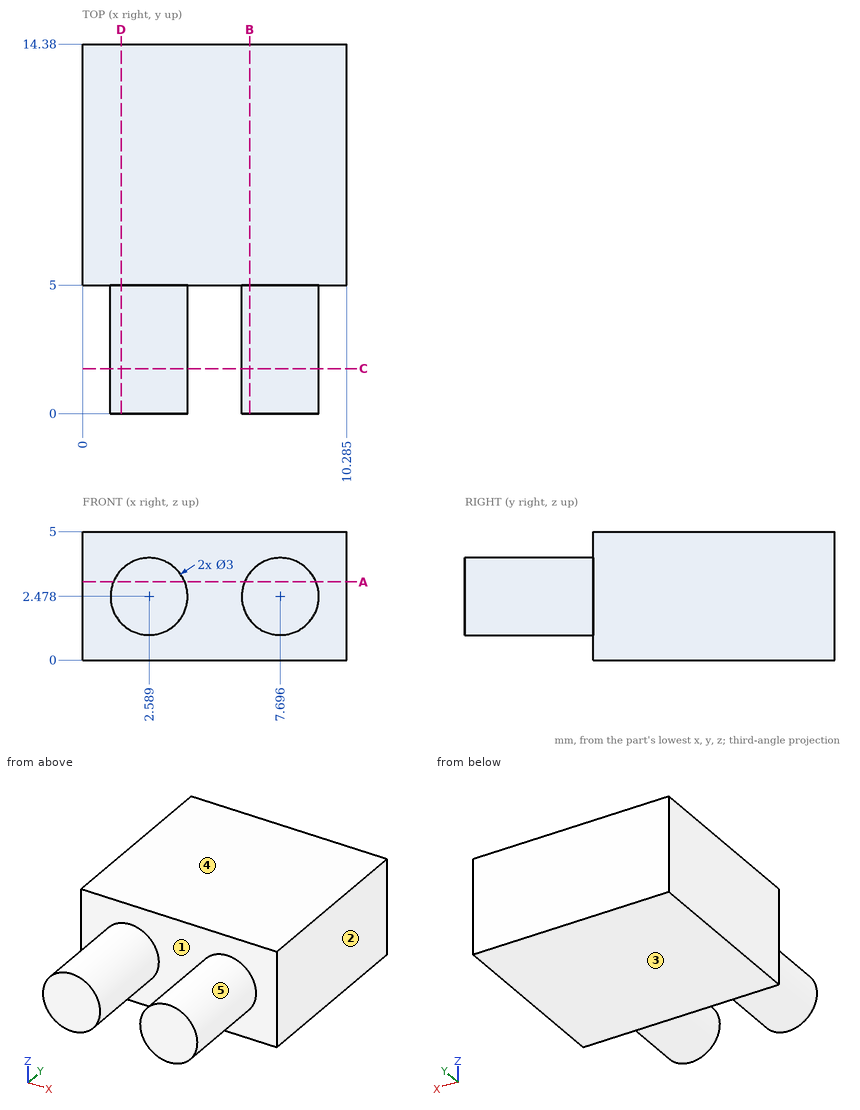
Could you check a few things on this drawing? It's one solid part, dimensions in mm from its lowest x, y, z. A direction names the side the tool comes from. Coordinates: 2 decimals unless noted, no trailing zeros. Loops run counter-clockwise (first coordinate to the right, second up) from the corner with the lowest first, then second, coordinate; pieces in that order, holes last. Notation, with made-up numbers: (16, 35.5) - (57, 35.5) arc R23 ccw to (57, 43.5) - close; hole circle Ø3 at (31, 59.25). An arc over 180 degrees is marked (long way). Return JSON: item names as keys, results as strings. Group by question number.
Item 1: If we section it at D-D on x = 1.5: Write out the boundary of the cut face in (y, z).
Item 2: I need wall thicknesses on line 1 (Y direction, x = 4.75, z = 3); line 2 (X direction, y = 4.25, z = 3.2) (1 decimal); line 3 (Z direction, x = 2, y = 4). Which ranges of each line are inside material? Lowest first, please. Write a range as from..to.
Item 3: If we section it at C-C on y = 1.75: Write out the boundary of the cut face in (x, z) (1 decimal).
Item 4: If we section it at B-B on x = 6.5: Write out the boundary of the cut face in (y, z).
Item 5: If we section it at A-A on z = 3.05: Write out the boundary of the cut face in (x, y) (1 decimal).
Item 6: On a 3-axis mill with a long thin cutter (end or side, diameter ignored), from which of +Z, -Z, +X, -X, +Y, -Y can I reach the whole of each face in a straight line? I mean the marked faces 4 and 5. Say none if no direction works.
Item 7: We'd pull the mould along X, two halves only. Please class the marked faces 1, 2 and 3: +X half, -X half, draft (parallel to the pull), parting line (faces both ways), or undercut.
Calculated:
{
 "1": {"outline": "(0, 1.45) - (5, 1.45) - (5, 0) - (14.38, 0) - (14.38, 5) - (5, 5) - (5, 3.51) - (0, 3.51) - close"},
 "2": {"line 1": "y = 5..14.38", "line 2": "x = 1.3..3.9, 6.4..9", "line 3": "z = 1.1..3.86"},
 "3": {"outline": "circle Ø3 at (2.6, 2.5); circle Ø3 at (7.7, 2.5)"},
 "4": {"outline": "(0, 1.57) - (5, 1.57) - (5, 0) - (14.38, 0) - (14.38, 5) - (5, 5) - (5, 3.38) - (0, 3.38) - close"},
 "5": {"outline": "(0, 5) - (1.2, 5) - (1.2, 0) - (4, 0) - (4, 5) - (6.3, 5) - (6.3, 0) - (9.1, 0) - (9.1, 5) - (10.3, 5) - (10.3, 14.4) - (0, 14.4) - close"},
 "6": {"face 4": "+Z, +X, -X, +Y, -Y", "face 5": "-Y"},
 "7": {"face 1": "undercut", "face 2": "+X half", "face 3": "draft"}
}
